```python
from build123d import *

# Parameters (mm, degrees)
F0_W     = 19
F0_H     = 19
F0_W_2   = 14
F0_H_2   = 14
F1_DEPTH = 4
F2_W     = 3
F2_H     = 4
F3_DEPTH = 0.5
F5_DEPTH = 3
F6_W     = 3
F6_H     = 4
F7_DEPTH = 0.5
F9_DEPTH = 3


with BuildPart() as f1:
    # F0 (on Top) → F1 (new body)
    with BuildSketch(Plane.XY):
        Rectangle(F0_W, F0_H)
        Rectangle(F0_W_2, F0_H_2, mode=Mode.SUBTRACT)
    extrude(amount=F1_DEPTH)

    # F2 (on face) → F3 (join)
    with BuildSketch(Plane.YZ.offset(-7)):
        with Locations((0, 2)):
            Rectangle(F2_W, F2_H)
    extrude(amount=F3_DEPTH)

    # F4 (on face) → F5 (cut, through all)
    with BuildSketch(Plane.XZ.offset(1.5)):
        Polygon((-6.5, 4), (-7, 4), (-6.5, 0), align=None)
    extrude(amount=-F5_DEPTH, mode=Mode.SUBTRACT)

    # F6 (on face) → F7 (join)
    with BuildSketch(Plane(origin=(7, 0, 0), x_dir=(0, -1, 0), z_dir=(-1, 0, 0))):
        with Locations((0, 2)):
            Rectangle(F6_W, F6_H)
    extrude(amount=F7_DEPTH)

    # F8 (on face) → F9 (cut, through all)
    with BuildSketch(Plane.XZ.offset(1.5)):
        Polygon((6.5, 4), (6.5, 0), (7, 4), align=None)
    extrude(amount=-F9_DEPTH, mode=Mode.SUBTRACT)


solid = f1.part
```
Could you check a few things on this model? Use its own coordinates, in mm. A direction names the side the tool comes from. Round coordinates to 2 decimals unless told otherwise and drop trailing zeros. Write each loop counter-clockwise with the first axis right and the second up, starting at its lowest first coordinate (ties: lowest second). Pieces come first, ordered by that corner, then holes.
(1) Suppose I cut it at A-A on y = 1. Write out the boundary of the cut face in (x, z).
Findings below:
outline: (-9.5, 0) - (-6.5, 0) - (-7, 4) - (-9.5, 4) - close; (6.5, 0) - (9.5, 0) - (9.5, 4) - (7, 4) - close
(2) Thinking about a two-plate mould opening in Y: for faces 1 (the face through (0, -9.5, 2)), 2 (the face through (-7, -4, 2)), 3 (the face through (0, 9.5, 2)), 4 (the face through (-9.5, 0, 2)), which applies, +Y half, -Y half, draft (parallel to the pull), parting line (faces both ways), or undercut?
Findings below:
face 1: -Y half
face 2: undercut
face 3: +Y half
face 4: draft
(3) Suppose I cut it at C-C on z = 2.8. Write out the boundary of the cut face in (x, y).
Findings below:
outline: (-9.5, -9.5) - (9.5, -9.5) - (9.5, 9.5) - (-9.5, 9.5) - close; hole (-7, -7) - (7, -7) - (7, -1.5) - (6.85, -1.5) - (6.85, 1.5) - (7, 1.5) - (7, 7) - (-7, 7) - (-7, 1.5) - (-6.85, 1.5) - (-6.85, -1.5) - (-7, -1.5) - close
(4) Suppose I cut it at D-D on z = 0.5. Write out the boundary of the cut face in (x, y).
Findings below:
outline: (-9.5, -9.5) - (9.5, -9.5) - (9.5, 9.5) - (-9.5, 9.5) - close; hole (-7, -7) - (7, -7) - (7, -1.5) - (6.56, -1.5) - (6.56, 1.5) - (7, 1.5) - (7, 7) - (-7, 7) - (-7, 1.5) - (-6.56, 1.5) - (-6.56, -1.5) - (-7, -1.5) - close
(5) Which directions (+Z, -Z, +X, -X, +Y, -Y) give clear straight access to the entire face, cutting with the end or side of a thin tool? Please do faces 5 (the face through (0, -7, 2)), 6 (the face through (6.746, -0.021, 1.972)), 7 (the face through (8, 0, 4)).
Findings below:
face 5: +Z, -Z
face 6: +Z
face 7: +Z, +X, -X, +Y, -Y
(6) Suppose I cut it at B-B on x = -3.75. Write out the boundary of the cut face in (y, z).
Findings below:
outline: (-9.5, 0) - (-7, 0) - (-7, 4) - (-9.5, 4) - close; (7, 0) - (9.5, 0) - (9.5, 4) - (7, 4) - close
(7) If I drill on probe 1 along Y at (x, z) = (3.5, 3); probe 2 along X at (y, z) = (-0.75, 1.45), over which ranges is the centre line in solid material (lowest first)?
Findings below:
probe 1: y = -9.5 to -7, 7 to 9.5
probe 2: x = -9.5 to -6.68, 6.68 to 9.5
